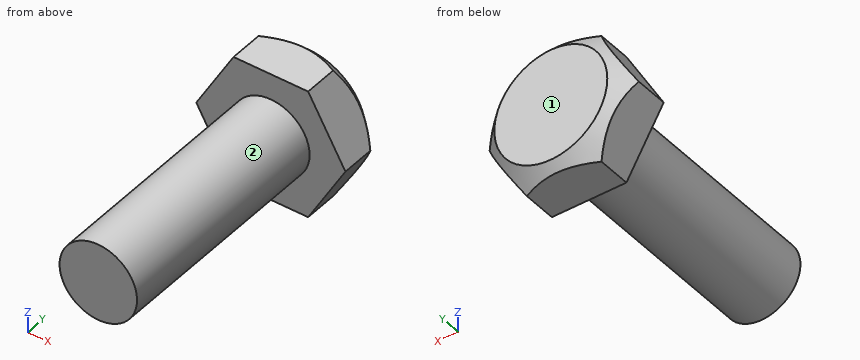
Autodesk Inventor part; units mm, degrees
ref_plane "YZ Plane" through (0, 0, 0) normal (1, 0, 0) x (0, 1, 0)
ref_plane "XZ Plane" through (0, 0, 0) normal (0, 1, 0) x (-1, 0, 0)
ref_plane "XY Plane" through (0, 0, 0) normal (0, 0, 1) x (1, 0, 0)
sketch "Boceto1" plane through (0, 0, 0) normal (0, 1, 0) x (-1, 0, 0)
  point P0 (0, 0)
sketch "Boceto2" plane through (0, 0, 0) normal (0, 1, 0) x (-1, 0, 0)
  line L0 (1.4434, -2.5) -> (-1.4434, -2.5)
  line L1 (-1.4434, -2.5) -> (-2.8868, 0)
  line L2 (-2.8868, 0) -> (-1.4434, 2.5)
  line L3 (-1.4434, 2.5) -> (1.4434, 2.5)
  line L4 (1.4434, 2.5) -> (2.8868, 0)
  line L5 (2.8868, 0) -> (1.4434, -2.5)
  point P0 (0, 0)
  point P1 (0, 0)
  dimension "d0" = 5
extrude "Extrusión1" add sketch "Boceto2" along normal blind 2
sketch "Boceto3" plane through (0, 0, 0) normal (0, -1, 0) x (1, 0, 0)
  circle A0 centre (0, 0) radius 1.5
  dimension "d3" = 3
extrude "Extrusión2" add sketch "Boceto3" along normal blind 9
sketch "Boceto4" plane through (0, 0, 0) normal (0, 0, 1) x (1, 0, 0)
  line L0 (-2.8868, 0) -> (-2.8868, 2)
  line L1 (-2.8868, 1.3) -> (-2.8868, 2)
  line L2 (-2.8868, 2) -> (-2.1868, 2)
  line L3 (-2.8868, 2) -> (-1.4434, 2)
  line L4 (-2.8868, 1.3) -> (-2.1868, 2)
  line L5 (0, -11.2) -> (0, 4.2)
  point P0 (0, 0)
  dimension "d6" = 0.7
  dimension "d7" = 0.7
revolve "Revolución1" cut sketch "Boceto4" angle 360 about axis through (0, -10, 0) along (0, 1, 0)
thread "Rosca1"
properties part number "Tornillo" material "Acero inoxidable"
Input: part model. Units: mm. Frame: model coordinates. Face numbers are marked on the shaded views. A direction names the side the tool comes from. Coordinates: 2 decimals unless noted, no trailing zeros. Write each loop counter-clockwise with the first axis right and the second up, starting at its lowest first coordinate (ties: lowest second). Pieces come first, ordered by that corner, then holes. Notation, with made-up numbers: M -9,84.5 L 31,84.5 A15 cw 31,96.5 Z; hole C 36.25,47 d8. An arc over 180 degrees is marked long. Use one line per item in the form item = value.
Q1. Material intervals for probe 1 along Z at (x, y) = (-0.4, -6); probe 2 along Y at (x, z) = (-1.55, 1.2); probe 3 along X at (y, z) = (-3, -1.1), sorted ascending. Write a range as from..to.
Answer below:
probe_1 = -1.45..1.45
probe_2 = 0..2
probe_3 = -1.02..1.02
Q2. Set-up query: the marked faces 1 and 2. Return all of +Z, -Z, +X, -X, +Y, -Y with unobstructed straight access to the full face (end or side cutting, diameter ignored); none if empty.
Answer below:
face_1 = +Z, -Z, +X, -X, +Y
face_2 = -Y
Q3. Section A-A (x = 0). Return loops of the section in (y, z).
Answer below:
outline = M -9,-1.5 L 0,-1.5 L 0,-2.5 L 1.69,-2.5 L 2,-2.19 L 2,2.19 L 1.69,2.5 L 0,2.5 L 0,1.5 L -9,1.5 Z
Q4. Section B-B (y = 0.5). Return loops of the section in (x, z), plus the area to 3 significant figures.
Answer below:
outline = M -2.89,0 L -1.44,-2.5 L 1.44,-2.5 L 2.89,0 L 1.44,2.5 L -1.44,2.5 Z
area = 21.7 mm²
Q5. First-contact query: pin 1 (1 mm diameter, centred on x = -0.5, y = -2, fed in from +Z); pin 2 (1 mm diameter, centred on y = -3, z = -0.5, fed in from -X). Flat tips, straight axial feed; report the tip coordinate or a pass-through.
Answer below:
pin_1 = 1.5
pin_2 = -1.5
